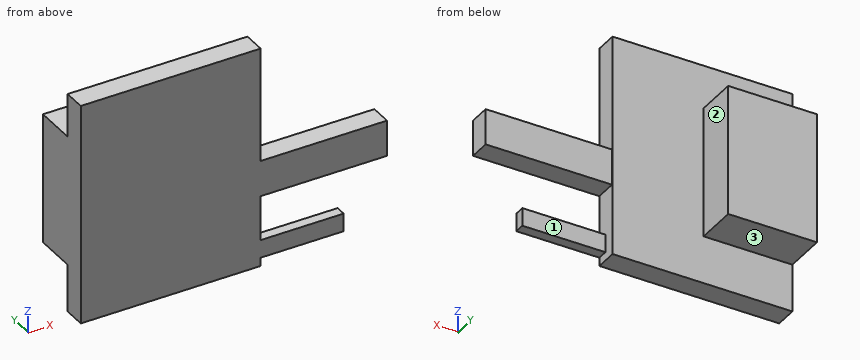
Autodesk Inventor part; units mm, degrees
ref_plane "YZ Plane" through (0, 0, 0) normal (1, 0, 0) x (0, 1, 0)
ref_plane "XZ Plane" through (0, 0, 0) normal (0, 1, 0) x (-1, 0, 0)
ref_plane "XY Plane" through (0, 0, 0) normal (0, 0, 1) x (1, 0, 0)
sketch "Sketch1" plane through (0, 0, 0) normal (0, 1, 0) x (-1, 0, 0)
  line L0 (-40.5, 50) -> (40.5, 50)
  line L1 (40.5, 50) -> (40.5, -50)
  line L2 (40.5, -50) -> (-40.5, -50)
  line L3 (-40.5, -50) -> (-40.5, 50)
  line L4 (-40.5, 50) -> (40.5, -50) construction
  line L5 (40.5, 50) -> (-40.5, -50) construction
  point P0 (0, 0)
  dimension "d0" = 81
  dimension "d1" = 100
extrude "Extrusion1" add sketch "Sketch1" along normal blind 28.7
sketch "Sketch2" plane through (40.5, 0, 50) normal (1, 0, 0) x (0, 0, -1)
  line L0 (100, 0) -> (0, 0)
  line L1 (67.9, 0) -> (67.9, 9.6)
  line L2 (67.9, 9.6) -> (51.7, 9.6)
  line L3 (51.7, 9.6) -> (51.7, 0)
  line L4 (51.7, 0) -> (67.9, 0)
  point P0 (50, 0)
  dimension "d5" = 9.6
  dimension "d6" = 16.2
extrude "Extrusion2" add sketch "Sketch2" along normal blind 56.9
sketch "Sketch3" plane through (40.5, 0, -50) normal (1, 0, 0) x (0, 0, -1)
  line L0 (-32.1, 0) -> (0, 0)
  line L1 (0, 0) -> (-3.8, 0)
  line L2 (-3.8, 0) -> (-3.8, 4.6)
  line L3 (-3.8, 4.6) -> (-11.9, 4.6)
  line L4 (-11.9, 4.6) -> (-11.9, 0)
  line L5 (-11.9, 0) -> (-3.8, 0)
  point P0 (-50, 0)
  dimension "d9" = 3.8
  dimension "d10" = 4.6
  dimension "d11" = 8.1
extrude "Extrusion3" add sketch "Sketch3" along normal blind 37.4
sketch "Sketch4" plane through (0, 28.7, 0) normal (0, 1, 0) x (1, 0, 0)
  line L0 (-40.5, 50) -> (-40.5, -50)
  line L1 (-40.5, -50) -> (-40.5, -30.4)
  line L2 (-40.5, -30.4) -> (-0.5, -30.4)
  line L3 (-0.5, -30.4) -> (-0.5, 28.5)
  line L4 (-0.5, 28.5) -> (-40.5, 28.5)
  line L5 (-40.5, 28.5) -> (-40.5, -30.4)
  line L6 (-40.5, -50) -> (40.5, -50)
  line L7 (-40.5, -50) -> (40.5, -50)
  line L8 (40.5, -50) -> (40.5, 50)
  line L9 (40.5, 38.1) -> (77.9, 38.1)
  line L10 (40.5, 50) -> (-40.5, 50)
  line L11 (40.5, 50) -> (-40.5, 50)
  line L12 (-40.5, 50) -> (-40.5, 28.5)
  point P0 (0, 0)
  dimension "d14" = 19.6
  dimension "d15" = 40
  dimension "d16" = 58.9
extrude "Extrusion4" cut sketch "Sketch4" against normal blind 18.7 contours L10 L8 L6 L0 L2 L3 L4
properties part number "NVidia"
The model under review builds one solid part; all positions refer to its coordinate system, in mm. Face numbers are marked on the shaded views. A direction names the side the tool comes from. Round coordinates to 2 decimals unless told otherwise and drop trailing zeros. Loops run counter-clockwise (first coordinate to the right, second up) from the corner with the lowest first, then second, coordinate; pieces in that order, holes last. Notation, with made-up numbers: (39, -14.75) -> (97, -14.75) arc R16 ccw to (97, -8.75) -> close; hole circle Ø3 at (43, -34). An arc over 180 degrees is marked (long way). Write item = value, one per line. Start each with the question number.
Item 1: For the marked faces 1, 2 and 3, list the 3-axis set-ups (+Z, -Z, +X, -X, +Y, -Y) from which the entire face can be reached by the end or side of a thin tool; tool diameter is ignored.
Item 2: To check wall thickness, follow L1, parallel to X at y = 14.25, z = 13.5; L2, parallel to Z at x = 42, y = 2; L3, parallel to Y at x = 21.5, z = -38.5. State the ranges of each line that lie inside material, in increasing order.
Item 3: Take a section at A-A on x = 54. Give the boundary of the cut face in (y, z).
Item 4: Take a section at C-C on y = 2.5. Give the boundary of the cut face in (x, z).
Item 5: Take a section at D-D on x = -26.5. Give the boundary of the cut face in (y, z).
Item 6: Insertion check: pin 1 (5.5 mm diameter, centred on y = 19.5, z = 2, fed in from +X); pin 2 (3 mm diameter, centred on x = 45.5, y = 9.5, fed in from -Z); pin 3 (1.4 mm diameter, centred on x = 60, y = 2.5, fed in from +Z). Each pin has a flat end and moves straight along its axis. Give the tip position at first contact, or say it passes through.
Item 7: Take a section at B-B on z = -14.5. Give the boundary of the cut face in (x, y), plus the area to 3 significant figures.
Result:
q1.face_1 = -Z, +X, +Y
q1.face_2 = +Z, -Z, +X, +Y
q1.face_3 = -Z, +X, -X, +Y
q2.L1 = -40.5 to -0.5
q2.L2 = -46.2 to -38.1, -17.9 to -1.7
q2.L3 = 0 to 10
q3.outline = (0, -46.2) -> (4.6, -46.2) -> (4.6, -38.1) -> (0, -38.1) -> close; (0, -17.9) -> (9.6, -17.9) -> (9.6, -1.7) -> (0, -1.7) -> close
q4.outline = (-40.5, -50) -> (40.5, -50) -> (40.5, -46.2) -> (77.9, -46.2) -> (77.9, -38.1) -> (40.5, -38.1) -> (40.5, -17.9) -> (97.4, -17.9) -> (97.4, -1.7) -> (40.5, -1.7) -> (40.5, 50) -> (-40.5, 50) -> close
q5.outline = (0, -50) -> (10, -50) -> (10, -28.5) -> (28.7, -28.5) -> (28.7, 30.4) -> (10, 30.4) -> (10, 50) -> (0, 50) -> close
q6.pin_1 = -0.5
q6.pin_2 = -17.9
q6.pin_3 = -1.7
q7.outline = (-40.5, 0) -> (97.4, 0) -> (97.4, 9.6) -> (40.5, 9.6) -> (40.5, 10) -> (-0.5, 10) -> (-0.5, 28.7) -> (-40.5, 28.7) -> close
q7.area = 2,100 mm²
